Build history of the part. All positions in model axes, mm. Face numbers are marked on the shaded views. Give positions to 0.01 mm unless a question says otherwise; leave off trailing zeros. Write each loop counter-clockwise with the first axis right and the second up, starting at its lowest first coordinate (ties: lowest second). Pieces come first, ordered by that corner, then holes. Notation, with made-up numbers: M -39,3 L -29,3 A12 ccw -29,13 Z; hole C 2,57 d8. An arc over 180 degrees is marked long. Return JSON: item names as keys, results as strings. Group by question number.
Q1. Band-saw the part on D-D, the plane z = 4.9. Give the cut face in (x, y), then the cut area to 3 significant figures.
Q2. Pull direction X, two halves, no side cores. Call the marked faces 1, 2 and 3: +X half, -X half, draft (parallel to the pull), parting line (faces both ways), or undercut.
Q3. Wall check: probe 1 along X at (y, z) = (-12, 3.7); probe 2 along Y at (x, z) = (-1, 1.05); probe 3 along Y at (x, z) = (20.5, 0.6). Give the ranges that are in metal, low to high.
Q4. Band-saw the part on C-C, the plane x = -7. Give the cut face in (y, z) (3 decimals).
Q5. Flat gauge pins, fed straight in: pin 1 Ø3 at (x, y) = (-20.78, -12) entering from +Z; pin 2 Ø1.5 at (y, z) = (-20.5, 5) entering from -X; pin 3 Ø3 at (y, z) = (19.5, 5) entering from +X. Where does each tip first touch, or does it go through?
Q6. Band-saw the part on A-A, the plane y = 0. Give the cut face in (x, z), then the cut area to 3 significant figures.
Q7. Band-saw the part on B-B, the plane x = 0. Give the cut face in (y, z).
from build123d import *

# Parameters (mm, degrees)
CYLINDER002_R     = 17.5
CYLINDER002_DEPTH = 10
CYLINDER_R        = 20
CYLINDER_DEPTH    = 3
CYLINDER003_R     = 1.7
CYLINDER003_DEPTH = 10
ARRAY001_COUNT    = 6
CYLINDER001_R     = 24
CYLINDER001_DEPTH = 6
CYLINDER004_R     = 4.7
CYLINDER004_DEPTH = 6
ARRAY_COUNT       = 6


with BuildPart() as cylinder002:
    # Cylinder002 → Cylinder002 (new body)
    with BuildSketch(Plane.XY):
        Circle(CYLINDER002_R)
    extrude(amount=CYLINDER002_DEPTH)


with BuildPart() as cylinder:
    # Cylinder → Cylinder (new body)
    with BuildSketch(Plane.XY.offset(3)):
        Circle(CYLINDER_R)
    extrude(amount=CYLINDER_DEPTH)


with BuildPart() as fusion001:
    # Cylinder003 → Cylinder003 (new body)
    with BuildSketch(Plane(origin=(0, -24, 0), x_dir=(1, 0, 0), z_dir=(0, 0, 1))):
        Circle(CYLINDER003_R)
    extrude(amount=CYLINDER003_DEPTH)

    # Array001: Fusion001 ×6 about axis
    array001_axis = Axis((0, 0, 0), (0, 0, 1))


with BuildPart() as fusion001_1:
    add(fusion001.part)
    for i in range(1, ARRAY001_COUNT):
        add(fusion001.part.rotate(array001_axis, i * 360 / ARRAY001_COUNT))

    # Fusion001: union Cylinder002, Cylinder
    add(cylinder002.part)
    add(cylinder.part)


with BuildPart() as cylinder001:
    # Cylinder001 → Cylinder001 (new body)
    with BuildSketch(Plane.XY):
        Circle(CYLINDER001_R)
    extrude(amount=CYLINDER001_DEPTH)


with BuildPart() as cut:
    # Cylinder004 → Cylinder004 (new body)
    with BuildSketch(Plane(origin=(0, -24, 0), x_dir=(1, 0, 0), z_dir=(0, 0, 1))):
        Circle(CYLINDER004_R)
    extrude(amount=CYLINDER004_DEPTH)

    # Array: Cut ×6 about axis
    array_axis = Axis((0, 0, 0), (0, 0, 1))


with BuildPart() as cut_1:
    add(cut.part)
    for i in range(1, ARRAY_COUNT):
        add(cut.part.rotate(array_axis, i * 360 / ARRAY_COUNT))

    # Fusion: union Cylinder001
    add(cylinder001.part)

    # Cut: cut Fusion001
    add(fusion001_1.part, mode=Mode.SUBTRACT)


solid = cut_1.part
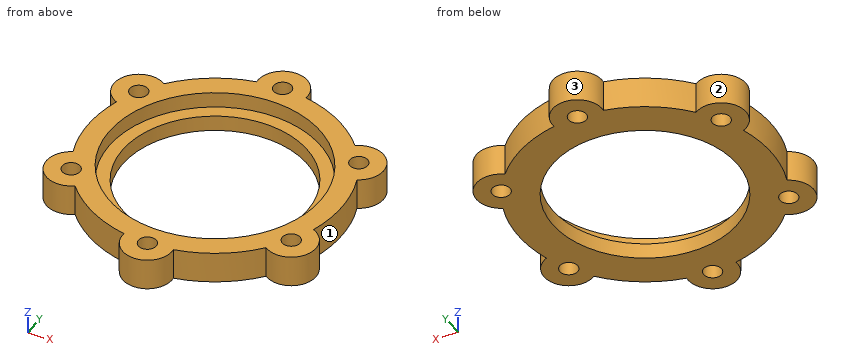
From the geometry:
{
 "1": {"outline": "M -22.72,-7.72 A4.7 ccw long -18.05,-15.82 A24 ccw -4.68,-23.54 A4.7 ccw long 4.68,-23.54 A24 ccw 18.05,-15.82 A4.7 ccw long 22.72,-7.72 A24 ccw 22.72,7.72 A4.7 ccw long 18.05,15.82 A24 ccw 4.68,23.54 A4.7 ccw long -4.68,23.54 A24 ccw -18.05,15.82 A4.7 ccw long -22.72,7.72 A24 ccw Z; hole C -20.78,-12 d3.4; hole C -20.78,12 d3.4; hole C 0,0 d40; hole C 0,-24 d3.4; hole C 0,24 d3.4; hole C 20.78,-12 d3.4; hole C 20.78,12 d3.4", "area": "715 mm^2"},
 "2": {"face 1": "+X half", "face 2": "undercut", "face 3": "parting line"},
 "3": {"probe 1": "x = -25.48 to -22.48, -19.08 to -16, 16 to 19.08, 22.48 to 25.48", "probe 2": "y = -28.59 to -25.37, -22.63 to -17.47, 17.47 to 22.63, 25.37 to 28.59", "probe 3": "y = -16.69 to -13.68, -10.32 to 10.32, 13.68 to 16.69"},
 "4": {"outline": "M -22.956,0 L -16.039,0 L -16.039,3 L -18.735,3 L -18.735,6 L -22.956,6 Z; M 16.039,0 L 22.956,0 L 22.956,6 L 18.735,6 L 18.735,3 L 16.039,3 Z"},
 "5": {"pin 1": "passes through", "pin 2": "stops at x = -13.64", "pin 3": "stops at x = 15.87"},
 "6": {"outline": "M -24,0 L -17.5,0 L -17.5,3 L -20,3 L -20,6 L -24,6 Z; M 17.5,0 L 24,0 L 24,6 L 20,6 L 20,3 L 17.5,3 Z", "area": "63.0 mm^2"},
 "7": {"outline": "M -28.7,0 L -25.7,0 L -25.7,6 L -28.7,6 Z; M -22.3,0 L -17.5,0 L -17.5,3 L -20,3 L -20,6 L -22.3,6 Z; M 17.5,0 L 22.3,0 L 22.3,6 L 20,6 L 20,3 L 17.5,3 Z; M 25.7,0 L 28.7,0 L 28.7,6 L 25.7,6 Z"}
}
